Source: CAD feature listing. Evaluate the final solid. Frame: model axes, mm. A direction names the side the tool comes from. Round coordinates to 2 decimals unless told otherwise and drop trailing zeros. Order: outer loops, then holes, each group sorted by start corner. A loop starts at its lowest first (then second) coordinate and runs counter-clockwise, first axis right, second up. Notation, with made-up numbers: (-30, 52.25) -> (-8, 52.25) arc R18 ccw to (-8, 60.25) -> close; hole circle Ø3 at (-12.75, 42). An arc over 180 degrees is marked (long way). Use a Markdown table: item, result. Add a question column.
```python
from build123d import *

# Parameters (mm, degrees)
SKICA1_W                 = 54.6
SKICA1_H                 = 54.6
P_IDAT_VYSUNUT_M2_DEPTH  = 3
SKICA5_W                 = 5
SKICA5_H                 = 24.8
SKICA5_W_2               = 54.6
SKICA5_H_2               = 5
ODEBRAT_VYSUNUT_M3_DEPTH = 1
SKICA14_W                = 52.6
SKICA14_H                = 1
P_IDAT_VYSUNUT_M9_DEPTH  = 15
SKICA17_R                = 2
ODEBRAT_VYSUNUT_M8_DEPTH = 7
SKICA19_W                = 7.8
SKICA19_H                = 7.8
P_IDAT_VYSUNUT_M10_DEPTH = 18
SKICA20_R                = 2.4
ODEBRAT_VYSUNUT_M9_DEPTH = 1.7
ZAOBLIT1_R               = 3


with BuildPart() as part:
    # Skica1 → Přidat vysunutím2 (new body)
    with BuildSketch(Plane.XY):
        Rectangle(SKICA1_W, SKICA1_H)
    extrude(amount=P_IDAT_VYSUNUT_M2_DEPTH)

    # Skica5 → Odebrat vysunutím3 (cut)
    with BuildSketch(Plane(origin=(0, 0, 0), x_dir=(-1, 0, 0), z_dir=(0, 0, -1))):
        with Locations((0, 14.9)):
            Rectangle(SKICA5_W, SKICA5_H)
        Rectangle(SKICA5_W_2, SKICA5_H_2)
        with Locations((0, -14.9)):
            Rectangle(SKICA5_W, SKICA5_H)
    extrude(amount=-ODEBRAT_VYSUNUT_M3_DEPTH, mode=Mode.SUBTRACT)

    # Skica14 → Přidat vysunutím9 (add)
    with BuildSketch(Plane.XY.offset(3)):
        Polygon((27.3, 27.3), (-27.3, 27.3), (-27.3, -27.3), (-26.3, -27.3), (-26.3, -26.3), (-26.3, 26.3), (26.3, 26.3), (26.3, -26.3), (26.3, -27.3), (27.3, -27.3), align=None)
        with Locations((0, -26.8)):
            Rectangle(SKICA14_W, SKICA14_H)
    extrude(amount=P_IDAT_VYSUNUT_M9_DEPTH)

    # Skica17 → Odebrat vysunutím8 (cut)
    with BuildSketch(Plane(origin=(0, 0, 1), x_dir=(-1, 0, 0), z_dir=(0, 0, -1))):
        with Locations((-20.3, 0)):
            Circle(SKICA17_R)
        with Locations((20.3, 0)):
            Circle(SKICA17_R)
        with Locations((0, 20.3)):
            Circle(SKICA17_R)
        with Locations((0, -20.3)):
            Circle(SKICA17_R)
    extrude(amount=-ODEBRAT_VYSUNUT_M8_DEPTH, mode=Mode.SUBTRACT)

    # Skica19 → Přidat vysunutím10 (add)
    with BuildSketch(Plane(origin=(0, 0, 0), x_dir=(-1, 0, 0), z_dir=(0, 0, -1))):
        with Locations((-23.4, 23.4)):
            Rectangle(SKICA19_W, SKICA19_H)
        with Locations((23.4, 23.4)):
            Rectangle(SKICA19_W, SKICA19_H)
        with Locations((-23.4, -23.4)):
            Rectangle(SKICA19_W, SKICA19_H)
        with Locations((23.4, -23.4)):
            Rectangle(SKICA19_W, SKICA19_H)
    extrude(amount=-P_IDAT_VYSUNUT_M10_DEPTH)

    # Skica20 → Odebrat vysunutím9 (cut)
    with BuildSketch(Plane.XY.offset(18)):
        with Locations((-23.4, -23.4)):
            Circle(SKICA20_R)
        with Locations((-23.4, 23.4)):
            Circle(SKICA20_R)
        with Locations((23.400280565, 23.4)):
            Circle(SKICA20_R)
        with Locations((23.400280565, -23.4)):
            Circle(SKICA20_R)
    extrude(amount=-ODEBRAT_VYSUNUT_M9_DEPTH, mode=Mode.SUBTRACT)

    # Zaoblit1
    zaoblit1_edges = [part.edges().sort_by_distance(p)[0] for p in [
        (19.5, 19.5, 10.5),
        (-19.5, 19.5, 10.5),
        (19.5, -19.5, 10.5),
        (-19.5, -19.5, 10.5),
    ]]
    fillet(zaoblit1_edges, radius=ZAOBLIT1_R)


solid = part.part
```
1) Reachability of faces 1 (the flat face through (19.5, -24, 10)), 2 (the cylindrical face through (0.434, -22.252, 1.986)) from +Z, -Z, +X, -X, +Y, -Y: full face, straight path, thin tool, end or side. Return the list, or none.
2) Draft query along X for faces 3 (the flat face through (-24, -19.5, 10)), 4 (the flat face through (0, -27.3, 9)), 5 (the flat face through (27.3, 0, 9)). Return one class per face: pulls with the +X half, pulls with the -X half, needs draft (parallel to the pull), parting line crosses it, or undercut.
3) Section C-C on y = 0. Output: boundary loops of the cut face in (x, z), then the cut area to 3 significant figures.
4) Section A-A on z = 5.75. Output: boundary loops of the cut face in (x, y), then the cut area to 3 significant figures.
5) Line query: probe 1 along X at (y, z) = (23.5, 17.25); probe 2 along Y at (x, z) = (-5.5, 14.75). Output: solid intervals per line, ascending. Write a range as from..to.
6) Section D-D on x = 20.3. Output: boundary loops of the cut face in (y, z).
7) First-contact query: pin 1 Ø4 at (x, y) = (4, -6) entering from +Z; pin 2 Ø3 at (x, y) = (23.4, -23.4) entering from +Z. Flat tips, straight axial feed; report the tip coordinate or a pass-through.
8) Section B-B on x = -23.4. Output: boundary loops of the cut face in (y, z), then the cut area to 3 significant figures.
Conclusion:
| question | item | result |
|---|---|---|
| 1 | face 1 | +Z |
| 1 | face 2 | +Z, -Z |
| 2 | face 3 | undercut |
| 2 | face 4 | needs draft |
| 2 | face 5 | pulls with the +X half |
| 3 | outline | (-27.3, 1) -> (-22.3, 1) -> (-22.3, 3) -> (-26.3, 3) -> (-26.3, 18) -> (-27.3, 18) -> close; (-18.3, 1) -> (18.3, 1) -> (18.3, 3) -> (-18.3, 3) -> close; (22.3, 1) -> (27.3, 1) -> (27.3, 18) -> (26.3, 18) -> (26.3, 3) -> (22.3, 3) -> close |
| 3 | area | 123 mm^2 |
| 4 | outline | (-27.3, -27.3) -> (27.3, -27.3) -> (27.3, 27.3) -> (-27.3, 27.3) -> close; hole (-26.3, -19.5) -> (-22.5, -19.5) arc R3 cw to (-19.5, -22.5) -> (-19.5, -26.3) -> (19.5, -26.3) -> (19.5, -22.5) arc R3 cw to (22.5, -19.5) -> (26.3, -19.5) -> (26.3, 19.5) -> (22.5, 19.5) arc R3 cw to (19.5, 22.5) -> (19.5, 26.3) -> (-19.5, 26.3) -> (-19.5, 22.5) arc R3 cw to (-22.5, 19.5) -> (-26.3, 19.5) -> close |
| 4 | area | 392 mm^2 |
| 5 | probe 1 | x = -27.3..-25.8, -21..-19.5, 19.5..21, 25.8..27.3 |
| 5 | probe 2 | y = -27.3..-26.3, 26.3..27.3 |
| 6 | outline | (-27.3, 0) -> (-2.5, 0) -> (-2.5, 1) -> (-2, 1) -> (-2, 3) -> (-20.46, 3) -> (-20.46, 18) -> (-27.3, 18) -> close; (2, 1) -> (2.5, 1) -> (2.5, 0) -> (27.3, 0) -> (27.3, 18) -> (20.46, 18) -> (20.46, 3) -> (2, 3) -> close |
| 7 | pin 1 | stops at z = 3 |
| 7 | pin 2 | stops at z = 16.3 |
| 8 | outline | (-27.3, 0) -> (-2.5, 0) -> (-2.5, 1) -> (2.5, 1) -> (2.5, 0) -> (27.3, 0) -> (27.3, 18) -> (25.8, 18) -> (25.8, 16.3) -> (21, 16.3) -> (21, 18) -> (19.5, 18) -> (19.5, 3) -> (-19.5, 3) -> (-19.5, 18) -> (-21, 18) -> (-21, 16.3) -> (-25.8, 16.3) -> (-25.8, 18) -> (-27.3, 18) -> close |
| 8 | area | 376 mm^2 |
